from build123d import *

# Parameters (mm, degrees)
R_VOLUTION3_ANGLE                       = 30
ESQUISSE2_W                             = 5
ESQUISSE2_H                             = 32
R_VOLUTION4_ANGLE                       = 1
ESQUISSE3_W                             = 6
ESQUISSE3_H                             = 33
ENL_VEMENT_DE_MATI_RE_R_VOLUTION1_ANGLE = 1
ENL_V_MAT_EXTRU_1_DEPTH                 = 300
ESQUISSE5_R                             = 2.5
ENL_V_MAT_EXTRU_2_DEPTH                 = 300


with BuildPart() as part:
    # Esquisse1 → Révolution3 (revolve)
    with BuildSketch(Plane.XY):
        with BuildLine():
            Line((-50, -300), (50, -300))
            ThreePointArc((50, -300), (100.401716993, -296.811878507), (150, -287.298334621))
            Line((150, -287.298334621), (150, -239.47331922))
            Line((150, -239.47331922), (140, -239.47331922))
            Line((140, -239.47331922), (140, -279.47331922))
            ThreePointArc((140, -279.47331922), (95.306762763, -287.359390293), (50, -290))
            Line((50, -290), (-50, -290))
            ThreePointArc((-50, -290), (-95.306762763, -287.359390293), (-140, -279.47331922))
            Line((-140, -279.47331922), (-140, -239.47331922))
            Line((-140, -239.47331922), (-150, -239.47331922))
            Line((-150, -239.47331922), (-150, -287.298334621))
            ThreePointArc((-150, -287.298334621), (-100.401716993, -296.811878507), (-50, -300))
        make_face()
    revolve(axis=Axis((0, 0, 0), (1, 0, 0)), revolution_arc=R_VOLUTION3_ANGLE)

    # Esquisse2 → Révolution4 (revolve)
    with BuildSketch(Plane.XY):
        with Locations((-147.5, -258.47331922)):
            Rectangle(ESQUISSE2_W, ESQUISSE2_H)
        with Locations((147.5, -258.47331922)):
            Rectangle(ESQUISSE2_W, ESQUISSE2_H)
    revolve(axis=Axis((-163.497361966, 0, 0), (-1, 0, 0)), revolution_arc=R_VOLUTION4_ANGLE)

    # Esquisse3 → Enlèvement de matière-Révolution1 (revolve, cut)
    with BuildSketch(Plane(origin=(0, 0, 0), x_dir=(1, 0, 0), z_dir=(0, 0.5000000000000011, -0.8660254037844382))):
        with Locations((-147, 258.97331922)):
            Rectangle(ESQUISSE3_W, ESQUISSE3_H)
        with Locations((147, 258.97331922)):
            Rectangle(ESQUISSE3_W, ESQUISSE3_H)
    revolve(axis=Axis((-66.768740816, 0, 0), (-1, 0, 0)), revolution_arc=ENL_VEMENT_DE_MATI_RE_R_VOLUTION1_ANGLE, mode=Mode.SUBTRACT)

    # Esquisse4 → Enlèv. mat.-Extru.1 (cut)
    with BuildSketch(Plane.ZY.offset(150)):
        Polygon((0, -242.47331922), (4.27460179, -244.891772551), (4.231742917, -242.436389359), align=None)
    extrude(amount=-ENL_V_MAT_EXTRU_1_DEPTH, mode=Mode.SUBTRACT)

    # Esquisse5 → Enlèv. mat.-Extru.2 (cut)
    with BuildSketch(Plane.ZY.offset(150)):
        with Locations((-22.614300571, -258.482638314)):
            Circle(ESQUISSE5_R)
        with Locations((-109.656760374, -235.159681502)):
            Circle(ESQUISSE5_R)
    extrude(amount=-ENL_V_MAT_EXTRU_2_DEPTH, mode=Mode.SUBTRACT)


solid = part.part
Build history of the part. All positions in model axes, mm. A direction names the side the tool comes from. Coordinates: 2 decimals unless noted, no trailing zeros. Order: outer loops, then holes, each group sorted by start corner. A loop starts at its lowest first (then second) coordinate and runs counter-clockwise, first axis right, second up. Notation, with made-up numbers: (-38, -39) - (20, -39) arc R18 cw to (20, -28) - close; hole circle Ø7 at (-20.5, 75). An arc over 180 degrees is marked (long way). Put each result on its own line as item: value.
1. Probe line 1 along X through (y, z) = (-235, -100); line 2 along Y through (x, z) = (134.5, -14); line 3 along Y through (x, z) = (-27.5, -9.5). List the from-to ranges inside material, lowest first. Write a range as [from, to].
Answer sheet:
line 1: x = [-150, -140], [140, 150]
line 2: y = [-290.64, -280.39]
line 3: y = [-299.85, -289.84]
2. Drop flat-ended pins along their axis: P1, Ø6.5, axis at y = -258.48, z = -22.61, coming from the +X side; P2, Ø10, axis at x = -93, z = -62.5, coming from the +Y side; P3, Ø6, axis at x = 29.5, z = -123, coming from the -Y side; P4, Ø5, axis at x = 37, z = -111.5, coming from the +Y side. Give the stop position or say it passes through.
Answer sheet:
P1: stops at x = 150
P2: stops at y = -279.45
P3: stops at y = -274.95
P4: stops at y = -266.65
3. Pull direction X, two halves, no side cores. Call faces 3 (the face through (-147.042, -226.705, -125.665)), 4 (the face through (150, -256, -70)), 5 (the face through (-0.7, -280.4, -74)): pulls with the +X half, pulls with the -X half, needs draft (parallel to the pull), parting line crosses it, or undercut.
Answer sheet:
face 3: needs draft
face 4: pulls with the +X half
face 5: undercut
4. Saw through at A-A (y = -229). Write the cut outline in (x, z), and give its area (3 significant figures).
Answer sheet:
outline: (-150, -126.94) - (-144, -126.94) - (-144, -132.21) - (-140, -132.21) - (-140, -70.05) - (-150, -70.05) - close; (140, -132.21) - (144, -132.21) - (144, -126.94) - (150, -126.94) - (150, -70.05) - (140, -70.05) - close
area: 1,180 mm^2
5. Saw through at B-B (x = -27.5). Write the cut outline in (y, z).
Answer sheet:
outline: (-300, 0) arc R300 ccw to (-259.81, -150) - (-251.15, -145) arc R290 cw to (-290, 0) - close
6. Tool access for faces 1 (the face through (140, -252, -71)), 2 (the face through (-145.07, -231.54, -61.13)): list every direction of +Z, -Z, +X, -X, +Y, -Y with a clear straight run to the whole face (end or side of a thin tool).
Answer sheet:
face 1: +Z, +Y
face 2: +Z, +X, -X, +Y
